from build123d import *

# Parameters (mm, degrees)
SKETCH_1_R          = 33
SKETCH_1_R_2        = 2
SKETCH_1_R_3        = 13
EXTRUDE_1_DEPTH     = 3
CUT_EXTRUDE_1_DEPTH = 47.765371804


with BuildPart() as part:
    # 草图1 → 凸台-拉伸1 (new body)
    with BuildSketch(Plane.XY):
        Circle(SKETCH_1_R)
        with Locations((-20.506096654, 20.506096654)):
            Circle(SKETCH_1_R_2, mode=Mode.SUBTRACT)
        with Locations((20.506096654, 20.506096654)):
            Circle(SKETCH_1_R_2, mode=Mode.SUBTRACT)
        with Locations((20.506096654, -20.506096654)):
            Circle(SKETCH_1_R_2, mode=Mode.SUBTRACT)
        with Locations((-20.506096654, -20.506096654)):
            Circle(SKETCH_1_R_2, mode=Mode.SUBTRACT)
        with Locations((-12.374368671, 12.374368671)):
            Circle(SKETCH_1_R_2, mode=Mode.SUBTRACT)
        with Locations((12.374368671, 12.374368671)):
            Circle(SKETCH_1_R_2, mode=Mode.SUBTRACT)
        with Locations((12.374368671, -12.374368671)):
            Circle(SKETCH_1_R_2, mode=Mode.SUBTRACT)
        with Locations((-12.374368671, -12.374368671)):
            Circle(SKETCH_1_R_2, mode=Mode.SUBTRACT)
        Circle(SKETCH_1_R_3, mode=Mode.SUBTRACT)
    extrude(amount=EXTRUDE_1_DEPTH)

    # 草图2 → 切除-拉伸1 (cut, through all)
    with BuildSketch(Plane.XY.offset(3)):
        with BuildLine():
            Line((-7.757359313, 16.242640687), (-15.096438919, 23.581720293))
            ThreePointArc((-15.096438919, 23.581720293), (0, 28), (15.096438919, 23.581720293))
            Line((15.096438919, 23.581720293), (7.757359313, 16.242640687))
            ThreePointArc((7.757359313, 16.242640687), (0, 18), (-7.757359313, 16.242640687))
        make_face()
        with BuildLine():
            Line((16.242640687, 7.757359313), (23.581720293, 15.096438919))
            ThreePointArc((23.581720293, 15.096438919), (28, 0), (23.581720293, -15.096438919))
            Line((23.581720293, -15.096438919), (16.242640687, -7.757359313))
            ThreePointArc((16.242640687, -7.757359313), (18, 0), (16.242640687, 7.757359313))
        make_face()
        with BuildLine():
            Line((7.757359313, -16.242640687), (15.096438919, -23.581720293))
            ThreePointArc((15.096438919, -23.581720293), (0, -28), (-15.096438919, -23.581720293))
            Line((-15.096438919, -23.581720293), (-7.757359313, -16.242640687))
            ThreePointArc((-7.757359313, -16.242640687), (0, -18), (7.757359313, -16.242640687))
        make_face()
        with BuildLine():
            Line((-16.242640687, -7.757359313), (-23.581720293, -15.096438919))
            ThreePointArc((-23.581720293, -15.096438919), (-28, 0), (-23.581720293, 15.096438919))
            Line((-23.581720293, 15.096438919), (-16.242640687, 7.757359313))
            ThreePointArc((-16.242640687, 7.757359313), (-18, 0), (-16.242640687, -7.757359313))
        make_face()
    extrude(amount=-CUT_EXTRUDE_1_DEPTH, mode=Mode.SUBTRACT)


solid = part.part
Source: CAD feature listing. Evaluate the final solid. Frame: model axes, mm. Give positions to 0.01 mm unless a question says otherwise; leave off trailing zeros. Write each loop counter-clockwise with the first axis right and the second up, starting at its lowest first coordinate (ties: lowest second). Pieces come first, ordered by that corner, then holes. Notation, with made-up numbers: M -39,36 L -26,36 A26 cw -26,73 Z; hole C 80.25,16 d1. An arc over 180 degrees is marked long. Return JSON: item names as keys, results as strings. Group by question number.
1) Cut plane D-D, the plane x = 12. Output: boundary loops of the cut face in (y, z), then the cut area to 3 significant figures.
2) Cut plane C-C, the plane z = 2.3. Give the number of separate pieces and of enclosed holes in the cut face, then the cut area to 3 significant figures.
3) Draft query along X for faces 1 (the face through (-10.316, -7.91, 1.479)), 2 (the face through (0, -14, 0)). Return one class per face: released by +X, released by -X, zero draft, split by the parting line, or undercut.
4) Ray query, L1, parallel to X at y = 0.5, z = 2.5; L2, parallel to X at y = -3, z = 0.65; L3, parallel to Y at x = 8.5, z = 0.5. Return the intervals inside material, ascending.
5) Cut plane A-A, the plane y = 0. Output: boundary loops of the cut face in (x, z).
6) First-contact query: pin 1 Ø1 at (y, z) = (-3, 2) entering from -X; pin 2 Ø1.5 at (y, z) = (23.5, 2) entering from -X; pin 3 Ø1 at (x, z) = (-23.5, 2.5) entering from +Y. Flat tips, straight axial feed; report the tip coordinate or a pass-through.
Data:
{
 "1": {"outline": "M -30.74,0 L -25.3,0 L -25.3,3 L -30.74,3 Z; M -20.49,0 L -14.34,0 L -14.34,3 L -20.49,3 Z; M -10.41,0 L -5,0 L -5,3 L -10.41,3 Z; M 5,0 L 10.41,0 L 10.41,3 L 5,3 Z; M 14.34,0 L 20.49,0 L 20.49,3 L 14.34,3 Z; M 25.3,0 L 30.74,0 L 30.74,3 L 25.3,3 Z", "area": "102 mm²"},
 "2": {"separate pieces": "1", "enclosed holes": "13", "area": "1,830 mm²"},
 "3": {"face 1": "undercut", "face 2": "zero draft"},
 "4": {"L1": "x = -33 to -28, -17.99 to -12.99, 12.99 to 17.99, 28 to 33", "L2": "x = -32.86 to -27.84, -17.75 to -12.65, 12.65 to 17.75, 27.84 to 32.86", "L3": "y = -31.89 to -26.68, -16.99 to -9.84, 9.84 to 16.99, 26.68 to 31.89"},
 "5": {"outline": "M -33,0 L -28,0 L -28,3 L -33,3 Z; M -18,0 L -13,0 L -13,3 L -18,3 Z; M 13,0 L 18,0 L 18,3 L 13,3 Z; M 28,0 L 33,0 L 33,3 L 28,3 Z"},
 "6": {"pin 1": "stops at x = -32.91", "pin 2": "stops at x = -23.9", "pin 3": "stops at y = 23.66"}
}
